Work out the finished part from the listing and answer in its coordinate system (mm). Give positions to 0.01 mm unless a question says otherwise; leave off trailing zeros. Order: outer loops, then holes, each group sorted by start corner. A loop starts at its lowest first (then second) coordinate and runs counter-clockwise, first axis right, second up.
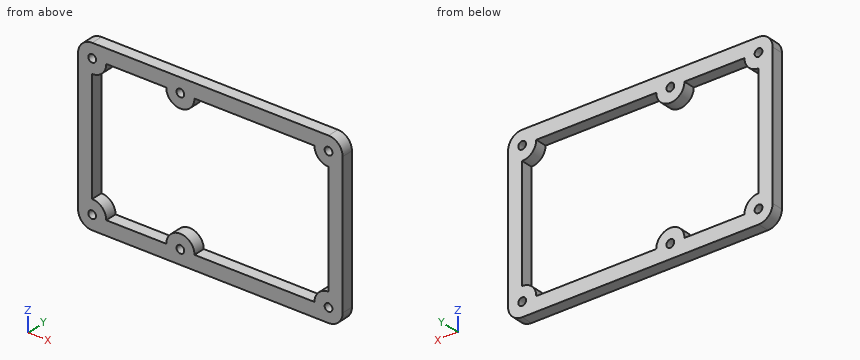
```python
from build123d import *

# Parameters (mm, degrees)
SKETCH_1_R      = 1.65
EXTRUDE_1_DEPTH = 5


with BuildPart() as part:
    # 草图1 → 凸台-拉伸1 (new body)
    with BuildSketch(Plane(origin=(0, 0, 0), x_dir=(1, 0, 0), z_dir=(0, 1, 0))):
        with BuildLine():
            Line((-62.785835682, 53.136639907), (-62.785835682, -6.863360093))
            ThreePointArc((-62.785835682, -6.863360093), (-61.028476369, -11.10600078), (-56.785835682, -12.863360093))
            Line((-56.785835682, -12.863360093), (43.714164318, -12.863360093))
            ThreePointArc((43.714164318, -12.863360093), (47.956805005, -11.10600078), (49.714164318, -6.863360093))
            Line((49.714164318, -6.863360093), (49.714164318, 53.136639907))
            ThreePointArc((49.714164318, 53.136639907), (47.956805005, 57.379280594), (43.714164318, 59.136639907))
            Line((43.714164318, 59.136639907), (-56.785835682, 59.136639907))
            ThreePointArc((-56.785835682, 59.136639907), (-61.028476369, 57.379280594), (-62.785835682, 53.136639907))
        make_face()
        with Locations(Location((-56.785835682, 53.136639907, 0), (0, 0, 270))):
            Circle(SKETCH_1_R, mode=Mode.SUBTRACT)
        with Locations(Location((-19.285835682, 53.136639907, 0), (0, 0, 270))):
            Circle(SKETCH_1_R, mode=Mode.SUBTRACT)
        with Locations(Location((43.714164318, 53.136639907, 0), (0, 0, 270))):
            Circle(SKETCH_1_R, mode=Mode.SUBTRACT)
        with Locations(Location((-56.785835682, -6.863360093, 0), (0, 0, 270))):
            Circle(SKETCH_1_R, mode=Mode.SUBTRACT)
        with Locations(Location((-19.285835682, -6.863360093, 0), (0, 0, 270))):
            Circle(SKETCH_1_R, mode=Mode.SUBTRACT)
        with Locations(Location((43.714164318, -6.863360093, 0), (0, 0, 270))):
            Circle(SKETCH_1_R, mode=Mode.SUBTRACT)
        with BuildLine():
            Line((-50.785835682, -6.863360093), (-25.285835682, -6.863360093))
            ThreePointArc((-25.285835682, -6.863360093), (-19.285835682, -0.863360093), (-13.285835682, -6.863360093))
            Line((-13.285835682, -6.863360093), (37.714164318, -6.863360093))
            ThreePointArc((37.714164318, -6.863360093), (39.471523631, -2.620719406), (43.714164318, -0.863360093))
            Line((43.714164318, -0.863360093), (43.714164318, 47.136639907))
            ThreePointArc((43.714164318, 47.136639907), (39.471523631, 48.89399922), (37.714164318, 53.136639907))
            Line((37.714164318, 53.136639907), (-13.285835682, 53.136639907))
            ThreePointArc((-13.285835682, 53.136639907), (-19.285835682, 47.136639907), (-25.285835682, 53.136639907))
            Line((-25.285835682, 53.136639907), (-50.785835682, 53.136639907))
            ThreePointArc((-50.785835682, 53.136639907), (-52.543194995, 48.89399922), (-56.785835682, 47.136639907))
            Line((-56.785835682, 47.136639907), (-56.785835682, -0.863360093))
            ThreePointArc((-56.785835682, -0.863360093), (-52.543194995, -2.620719406), (-50.785835682, -6.863360093))
        make_face(mode=Mode.SUBTRACT)
    extrude(amount=EXTRUDE_1_DEPTH)


solid = part.part
```
1. The part is cut by section A-A (z = -44). Write down the section's boundary in (x, y).
Findings below:
outline: (-62.79, 0) - (-56.79, 0) - (-56.79, 5) - (-62.79, 5) - close; (43.71, 0) - (49.71, 0) - (49.71, 5) - (43.71, 5) - close
2. The part is cut by section B-B (x = 2.5). Write down the section's boundary in (y, z), then the cut area to 3 significant figures.
Findings below:
outline: (0, -59.14) - (5, -59.14) - (5, -53.14) - (0, -53.14) - close; (0, 6.86) - (5, 6.86) - (5, 12.86) - (0, 12.86) - close
area: 60.0 mm2
3. The part is cut by section C-C (y = 1.8). Write down the section's boundary in (x, z).
Findings below:
outline: (-62.79, -53.14) arc R6 ccw to (-56.79, -59.14) - (43.71, -59.14) arc R6 ccw to (49.71, -53.14) - (49.71, 6.86) arc R6 ccw to (43.71, 12.86) - (-56.79, 12.86) arc R6 ccw to (-62.79, 6.86) - close; hole circle Ø3.3 at (-56.79, -53.14); hole circle Ø3.3 at (-56.79, 6.86); hole (-56.79, -47.14) arc R6 cw to (-50.79, -53.14) - (-25.29, -53.14) arc R6 cw to (-13.29, -53.14) - (37.71, -53.14) arc R6 cw to (43.71, -47.14) - (43.71, 0.86) arc R6 cw to (37.71, 6.86) - (-13.29, 6.86) arc R6 cw to (-25.29, 6.86) - (-50.79, 6.86) arc R6 cw to (-56.79, 0.86) - close; hole circle Ø3.3 at (-19.29, -53.14); hole circle Ø3.3 at (-19.29, 6.86); hole circle Ø3.3 at (43.71, -53.14); hole circle Ø3.3 at (43.71, 6.86)
4. Straight lines are drawn through the part: probe 1 along Z at (x, y) = (43.5, 2.5); probe 2 along Z at (x, y) = (-32.5, 1.1); probe 3 along X at (y, z) = (0.6, -42). For each, find the intervals that lie inside material, in ascending order.
Findings below:
probe 1: z = -59.14 to -54.77, -51.5 to -47.14, 0.87 to 5.23, 8.5 to 12.86
probe 2: z = -59.14 to -53.14, 6.86 to 12.86
probe 3: x = -62.79 to -56.79, 43.71 to 49.71
